Could you check a few things on this model? Use its own coordinates, in mm. Give positions to 0.01 mm unless a question says otherwise; leave off trailing zeros. Write each loop counter-clockwise with the first axis right and the second up, starting at its lowest first coordinate (ties: lowest second). Pieces come first, ordered by that corner, then holes. Notation, with made-up numbers: (-0.5, 62) -> (28.5, 62) arc R22 cw to (28.5, 72) -> close; hole circle Ø6 at (35, 60). An arc over 180 degrees is marked (long way). One line per question, with ' | ' between items.
from build123d import *

# Parameters (mm, degrees)
SKETCH_1_W               = 65
SKETCH_1_H               = 76
EXTRUDE_1_DEPTH          = 3
FILLET_1_R               = 3
SKETCH_3_R               = 1.275
CUT_EXTRUDE_1_DEPTH      = 1
CUT_EXTRUDE_1_DEPTH_BACK = 4
SKETCH_6_R               = 2.025
CUT_EXTRUDE_3_DEPTH      = 10
HOLE_WIZARD_1_AT_2_COUNT = 2
HOLE_WIZARD_1_AT_2_PITCH = 15
HOLE_WIZARD_1_AT_3_COUNT = 2
HOLE_WIZARD_1_AT_3_PITCH = 21.360009363


with BuildPart() as part:
    # 草图1 → 凸台-拉伸1 (new body)
    with BuildSketch(Plane(origin=(0, 0, 0), x_dir=(1, 0, 0), z_dir=(0, 1, 0))):
        Rectangle(SKETCH_1_W, SKETCH_1_H)
    extrude(amount=EXTRUDE_1_DEPTH)

    # 圆角1
    fillet_1_edges = [part.edges().sort_by_distance(p)[0] for p in [
        (32.5, 1.5, 38),
        (-32.5, 1.5, 38),
        (-32.5, 1.5, -38),
        (32.5, 1.5, -38),
    ]]
    fillet(fillet_1_edges, radius=FILLET_1_R)

    # 草图3 → 切除-拉伸1 (cut, two sides)
    with BuildSketch(Plane(origin=(0, 3, 0), x_dir=(1, 0, 0), z_dir=(0, 1, 0))) as cut_extrude_1_sk:
        with Locations((28.7, -22)):
            Circle(SKETCH_3_R)
        with Locations((28.7, 22)):
            Circle(SKETCH_3_R)
        with Locations((-27.3, 33.75)):
            Circle(SKETCH_3_R)
        with Locations((-27.3, -33.75)):
            Circle(SKETCH_3_R)
    extrude(amount=CUT_EXTRUDE_1_DEPTH, mode=Mode.SUBTRACT)
    extrude(cut_extrude_1_sk.sketch, amount=-CUT_EXTRUDE_1_DEPTH_BACK, mode=Mode.SUBTRACT)

    # 草图6 → 切除-拉伸3 (cut)
    with BuildSketch(Plane(origin=(0, 3, 0), x_dir=(1, 0, 0), z_dir=(0, 1, 0))):
        with Locations((-27, -10)):
            Circle(SKETCH_6_R)
        with Locations((-12, -10)):
            Circle(SKETCH_6_R)
        with Locations((-19.5, 10)):
            Circle(SKETCH_6_R)
    extrude(amount=-CUT_EXTRUDE_3_DEPTH, mode=Mode.SUBTRACT)

    # 草图7 → 孔1 (revolve, cut)
    with BuildSketch(Plane(origin=(-12, 3, 10), x_dir=(0, 0, 1), z_dir=(1, 0, 0))):
        Polygon((0, 0), (0, 3), (2, 3), (2, 2), (4, 0), align=None)
    hole_wizard_1 = revolve(axis=Axis((-12, 9.445314094, 10), (0, -1, 0)), mode=Mode.SUBTRACT)

    # 孔1 at 2: 孔1 ×2
    with Locations(*[(-i * HOLE_WIZARD_1_AT_2_PITCH, 0, 0) for i in range(1, HOLE_WIZARD_1_AT_2_COUNT)]):
        add(hole_wizard_1, mode=Mode.SUBTRACT)

    # 孔1 at 3: 孔1 ×2
    with Locations(*[Vector(-0.351123442, 0, -0.936329178) * (i * HOLE_WIZARD_1_AT_3_PITCH) for i in range(1, HOLE_WIZARD_1_AT_3_COUNT)]):
        add(hole_wizard_1, mode=Mode.SUBTRACT)


solid = part.part
Q1. Imagine slicing it at B-B on z = 22. Please give me the cut outline in (x, y) (3 decimals).
Answer below:
outline: (-32.5, 0) -> (27.425, 0) -> (27.425, 3) -> (-32.5, 3) -> close; (29.975, 0) -> (32.5, 0) -> (32.5, 3) -> (29.975, 3) -> close
Q2. Imagine slicing it at A-A on x = -12. Please give me the cut outline in (y, z) (3 decimals).
Answer below:
outline: (0, -38) -> (3, -38) -> (3, 6) -> (1.025, 7.975) -> (0, 7.975) -> close; (0, 12.025) -> (1.025, 12.025) -> (3, 14) -> (3, 38) -> (0, 38) -> close
Q3. Imagine slicing it at D-D on z = -10. Please give me the cut outline in (x, y) (3 decimals).
Answer below:
outline: (-32.5, 0) -> (-21.525, 0) -> (-21.525, 1.025) -> (-23.5, 3) -> (-32.5, 3) -> close; (-17.475, 0) -> (32.5, 0) -> (32.5, 3) -> (-15.5, 3) -> (-17.475, 1.025) -> close
Q4. If I drill on line 1 along Z through (x, y) = (-27, 0.75) (3 decimals); line 2 along X through (y, z) = (0.65, 10) (3 decimals); line 3 along X through (y, z) = (0.8, -10) (3 decimals), over which ranges is the centre line in solid material (lowest first)?
Answer below:
line 1: z = -38 to -34.989, -32.511 to 7.975, 12.025 to 32.511, 34.989 to 38 | line 2: x = -32.5 to -29.025, -24.975 to -14.025, -9.975 to 32.5 | line 3: x = -32.5 to -21.525, -17.475 to 32.5
Q5. If we mould it in two halves opening along Z, with no side actions, what happens to faces 1 (the flat face through (0, 0, -1)), 2 (the flat face through (0, 1, -38)), 3 (the conical face through (-29.13, 1.15, 9.72))? For each: +Z half, -Z half, draft (parallel to the pull), parting line (faces both ways), or undercut.
Answer below:
face 1: draft | face 2: -Z half | face 3: undercut
Q6. Imagine slicing it at C-C on y = 1.6. Please give me the cut outline in (x, z) (3 decimals), and give its area (3 significant figures).
Answer below:
outline: (-32.5, -35) arc R3 ccw to (-29.5, -38) -> (29.5, -38) arc R3 ccw to (32.5, -35) -> (32.5, 35) arc R3 ccw to (29.5, 38) -> (-29.5, 38) arc R3 ccw to (-32.5, 35) -> close; hole circle Ø5.2 at (-27, 10); hole circle Ø2.55 at (-27.3, -33.75); hole circle Ø2.55 at (-27.3, 33.75); hole circle Ø5.2 at (-19.5, -10); hole circle Ø5.2 at (-12, 10); hole circle Ø2.55 at (28.7, -22); hole circle Ø2.55 at (28.7, 22) | area: 4,850 mm^2
Q7. Will this pin go through, and if not, where does the flat tip stop? pin 1 (4.5 mm diameter, centred on x = -19.5, z = -10, fed in from +Y).
Answer below:
pin 1: stops at y = 1.25
